from build123d import *

# Parameters (mm, degrees)
BOSS_EXTRU_1_DEPTH      = 5
ENL_V_MAT_EXTRU_1_REACH = 7
ESQUISSE2_R             = 2.5


with BuildPart() as part:
    # Esquisse1 → Boss.-Extru.1 (new body)
    with BuildSketch(Plane.XY):
        Polygon((0, 4.618802154), (-4, 2.309401077), (-4, -2.309401077), (0, -4.618802154), (4, -2.309401077), (4, 2.309401077), align=None)
    extrude(amount=BOSS_EXTRU_1_DEPTH)

    # Esquisse2 → Enlèv. mat.-Extru.1 (cut, up to next)
    with BuildSketch(Plane.XY.offset(5), mode=Mode.PRIVATE) as enl_v_mat_extru_1_sk1:
        Circle(ESQUISSE2_R)
    enl_v_mat_extru_1_tool1 = extrude(enl_v_mat_extru_1_sk1.sketch, amount=-ENL_V_MAT_EXTRU_1_REACH, mode=Mode.PRIVATE) & part.part
    add(enl_v_mat_extru_1_tool1.solids().sort_by_distance((0, 0, 5))[0], mode=Mode.SUBTRACT)

    # Esquisse4 → Enlèvement de matière-Révolution8 (revolve, cut)
    with BuildSketch(Plane(origin=(0, 0, 0), x_dir=(1, 0, 0), z_dir=(0, 1, 0))):
        Polygon((-8.330127019, -2.5), (-2.267949192, 1), (-9.330127019, 1), (-9.330127019, -6), (-2.267949192, -6), align=None)
    revolve(axis=Axis((0, 0, 0), (0, 0, 1)), mode=Mode.SUBTRACT)


solid = part.part
Geometry: final body of the model. Coordinates: model frame, mm. Round coordinates to 2 decimals unless told otherwise and drop trailing zeros. Order: outer loops, then holes, each group sorted by start corner. A loop starts at its lowest first (then second) coordinate and runs counter-clockwise, first axis right, second up.
Q1. Section A-A, the plane z = 2.2. Output: boundary loops of the cut face in (x, y), and give its area (3 significant figures).
Result sheet:
outline: (-4, -2.31) - (0, -4.62) - (4, -2.31) - (4, 2.31) - (0, 4.62) - (-4, 2.31) - close; hole circle Ø5 at (0, 0)
area: 35.8 mm2
Q2. Mould query, pull axis Y, two halves, no side actions, for faces 1 (the face through (0.01, 4.15, 4.913)), 2 (the face through (2, 2, 0)), 3 (the face through (-0.54, -2.44, 2.54)), 4 (the face through (-2.028, -3.448, 2.465)). Classes: released by +Y, released by -Y, zero draft, split by the parting line, or undercut.
Result sheet:
face 1: released by +Y
face 2: zero draft
face 3: undercut
face 4: released by -Y
Q3. Material intervals for probe 1 along Y at (x, z) = (2.25, 1.55); probe 2 along Y at (x, z) = (-1.5, 3.4); probe 3 along X at (y, z) = (0.25, 2.3), sorted ascending.
Result sheet:
probe 1: y = -3.32 to -1.09, 1.09 to 3.32
probe 2: y = -3.75 to -2, 2 to 3.75
probe 3: x = -4 to -2.49, 2.49 to 4
Q4. Pin query (flat end, axial travel): pin 1 (2 mm diameter, centred on y = -3.5, z = 2, fed in from -X); pin 2 (3 mm diameter, centred on x = 0, y = 0, fed in from -Z); pin 3 (1 mm diameter, centred on x = -1.5, y = 1.5, fed in from -Z). Return the tip coordinate at first contact, or that it passes through.
Result sheet:
pin 1: stops at x = -3.67
pin 2: passes through
pin 3: stops at z = 0
